from build123d import *

# Parameters (mm, degrees)
SKETCH1_R           = 0.5
SKETCH1_R_2         = 1.75
BOSS_EXTRUDE2_DEPTH = 1.6


with BuildPart() as part:
    # Sketch1 → Boss-Extrude2 (new body)
    with BuildSketch(Plane(origin=(0, 0, 0), x_dir=(1, 0, 0), z_dir=(0, 1, 0))):
        Polygon((78.84, 0), (0, 0), (0, -160), (120, -160), (120, 0), (91.12, 0), (91.12, 3.176), (78.84, 3.176), align=None)
        with Locations((86.9, -46.51)):
            Circle(SKETCH1_R, mode=Mode.SUBTRACT)
        with Locations((89.44, -46.51)):
            Circle(SKETCH1_R, mode=Mode.SUBTRACT)
        with Locations((91.98, -46.51)):
            Circle(SKETCH1_R, mode=Mode.SUBTRACT)
        with Locations((94.52, -46.51)):
            Circle(SKETCH1_R, mode=Mode.SUBTRACT)
        with Locations((97.06, -46.51)):
            Circle(SKETCH1_R, mode=Mode.SUBTRACT)
        with Locations((99.6, -46.51)):
            Circle(SKETCH1_R, mode=Mode.SUBTRACT)
        with Locations((102.14, -46.51)):
            Circle(SKETCH1_R, mode=Mode.SUBTRACT)
        with Locations((86.9, -31.27)):
            Circle(SKETCH1_R, mode=Mode.SUBTRACT)
        with Locations((89.44, -31.27)):
            Circle(SKETCH1_R, mode=Mode.SUBTRACT)
        with Locations((91.98, -31.27)):
            Circle(SKETCH1_R, mode=Mode.SUBTRACT)
        with Locations((94.52, -31.27)):
            Circle(SKETCH1_R, mode=Mode.SUBTRACT)
        with Locations((97.06, -31.27)):
            Circle(SKETCH1_R, mode=Mode.SUBTRACT)
        with Locations((99.6, -31.27)):
            Circle(SKETCH1_R, mode=Mode.SUBTRACT)
        with Locations((102.14, -31.27)):
            Circle(SKETCH1_R, mode=Mode.SUBTRACT)
        Polygon((63, -47.55), (63, -65), (15, -65), (15, -20), (63, -20), (63, -30.45), (58.372, -30.45), (58.372, -47.55), align=None, mode=Mode.SUBTRACT)
        with Locations((12, -82)):
            Circle(SKETCH1_R_2, mode=Mode.SUBTRACT)
        with Locations((12, -156)):
            Circle(SKETCH1_R_2, mode=Mode.SUBTRACT)
        with Locations((54, -82)):
            Circle(SKETCH1_R_2, mode=Mode.SUBTRACT)
        with Locations((39, -82)):
            Circle(SKETCH1_R_2, mode=Mode.SUBTRACT)
        with Locations((39, -156)):
            Circle(SKETCH1_R_2, mode=Mode.SUBTRACT)
        with Locations((54, -156)):
            Circle(SKETCH1_R_2, mode=Mode.SUBTRACT)
        with Locations((108, -82)):
            Circle(SKETCH1_R_2, mode=Mode.SUBTRACT)
        with Locations((108, -156)):
            Circle(SKETCH1_R_2, mode=Mode.SUBTRACT)
        with Locations((66, -82)):
            Circle(SKETCH1_R_2, mode=Mode.SUBTRACT)
        with Locations((81, -156)):
            Circle(SKETCH1_R_2, mode=Mode.SUBTRACT)
        with Locations((81, -82)):
            Circle(SKETCH1_R_2, mode=Mode.SUBTRACT)
        with Locations((66, -156)):
            Circle(SKETCH1_R_2, mode=Mode.SUBTRACT)
    extrude(amount=BOSS_EXTRUDE2_DEPTH)


solid = part.part
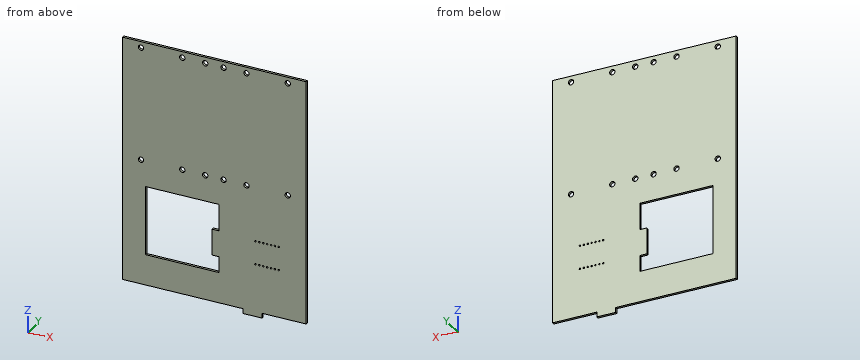
CAD build for the part. Positions are in the model's coordinates, mm. Give positions to 0.01 mm unless a question says otherwise; leave off trailing zeros. Order: outer loops, then holes, each group sorted by start corner. A loop starts at its lowest first (then second) coordinate and runs counter-clockwise, first axis right, second up. Notation, with made-up numbers: (-27.75, 87.25) - (21.25, 87.25) arc R4 ccw to (21.25, 92.25) - close; hole circle Ø7 at (-16, 27.25). An arc over 180 degrees is marked (long way). Answer in a Markdown table with one row per item.
1. Saw through at B-B, the plane z = 22. Give the cut face in (x, y).
Data:
| item | result |
|---|---|
| outline | (0, 0) - (15, 0) - (15, 1.6) - (0, 1.6) - close; (63, 0) - (120, 0) - (120, 1.6) - (63, 1.6) - close |
2. Saw through at C-C, the plane x = 66. Give the cut face in (y, z).
Data:
| item | result |
|---|---|
| outline | (0, 0) - (1.6, 0) - (1.6, 80.25) - (0, 80.25) - close; (0, 83.75) - (1.6, 83.75) - (1.6, 154.25) - (0, 154.25) - close; (0, 157.75) - (1.6, 157.75) - (1.6, 160) - (0, 160) - close |
3. Saw through at D-D, the plane y = 0.4. Count the separate pieces of the cut face and the enclosed holes in it, plus the area to 3 significant figures.
Data:
| item | result |
|---|---|
| separate pieces | 1 |
| enclosed holes | 27 |
| area | 17,000 mm² |
4. Flat gauge pins, fed straight in: pin 1 (5.5 mm diameter, centred on x = 81, z = 82, fed in from +Y); pin 2 (0.5 mm diameter, centred on x = 111.5, y = 0.5, fed in from -Z); pin 3 (3 mm diameter, centred on x = 12, z = 82, fed in from -Y); pin 4 (0.8 mm diameter, centred on y = 0.5, z = -2.5, fed in from +X). Where does each tip first touch, or does it go through?
Data:
| item | result |
|---|---|
| pin 1 | stops at y = 1.6 |
| pin 2 | stops at z = 0 |
| pin 3 | passes through |
| pin 4 | stops at x = 91.12 |
5. Saw through at A-A, the plane x = 47. Give the cut face in (y, z).
Data:
| item | result |
|---|---|
| outline | (0, 0) - (1.6, 0) - (1.6, 20) - (0, 20) - close; (0, 65) - (1.6, 65) - (1.6, 160) - (0, 160) - close |
6. Probe probe 1 along Z at (x, y) = (91.98, 1.05); probe 2 along Z at (x, y) = (54, 1); probe 3 along Z at (x, y) = (81, 0.95). List the from-to ranges inside material, lowest first. Write a range as [from, to].
Data:
| item | result |
|---|---|
| probe 1 | z = [0, 30.77], [31.77, 46.01], [47.01, 160] |
| probe 2 | z = [0, 20], [65, 80.25], [83.75, 154.25], [157.75, 160] |
| probe 3 | z = [-3.18, 80.25], [83.75, 154.25], [157.75, 160] |
